Could you check a few things on this model? Use its own coordinates, in mm. A direction names the side the tool comes from. Coordinates: 2 decimals unless noted, no trailing zeros. Write each loop counter-clockwise with the first axis right and the second up, starting at its lowest first coordinate (ties: lowest second). Pieces come first, ordered by that corner, then holes. Notation, with made-up numbers: M -3,17.25 L 16,17.25 A22 ccw 16,28.25 Z; hole C 43.25,31.25 d8. An arc over 180 degrees is marked long. Answer as CSV lines item,"result". Start each with the question number.
Item 1: I'm going to push flat-ended pins straight in: P1, Ø3, axis at y = 8.5, z = -17, coming from the +X side; P2, Ø4, axis at x = -25.5, z = 30.5, coming from the +Y side; P3, Ø1.7, axis at x = 20, z = 26.5, coming from the -Y side; P4, Ø3.5, axis at x = 31.5, z = -10, coming from the -Y side. Where does each tip first touch, or does it pass through?
Item 2: If I drill on line 1 along X through (y, z) = (10.4, 0); line 2 along Y through (x, z) = (-27, 0), over which ranges is the centre line in solid material (lowest first)? Write a range as [from, to].
Item 3: We'd pull the mould along Z, two halves only. Please class faces 1 (the flat face through (0, 11.7, -33)), 2 (the flat face through (-1, 16.5, -1)), 3 (the cylindrical face through (-5.077, 8.134, -38.668)): +Z half, -Z half, draft (parallel to the pull), parting line (faces both ways), or undercut.
Item 4: Suppose I cut it at A-A, the plane x = 0. Write out the boundary of the cut face in (y, z), and give its area (3 significant figures).
Item 5: Suppose I cut it at B-B, the plane y = 10.5. Write out the boundary of the cut face in (x, z).
Item 6: Suppose I cut it at D-D, the plane y = 4.75. Write out the boundary of the cut face in (x, z), and give its area (3 significant figures).
Item 7: On a 3-axis mill with a long thin cutter (end or side, diameter ignored), from which of +Z, -Z, +X, -X, +Y, -Y can I reach the whole of each face in a straight line? I mean faces 4 (the flat face through (11.4, 0, 34.5)), 5 (the flat face through (19, 11.7, 27)). Say none if no direction works.
Item 8: Suppose I cut it at C-C, the plane z = -2. Write out the boundary of the cut face in (x, y).
```python
from build123d import *

# Parameters (mm, degrees)
SKETCH1_R           = 39
SKETCH1_R_2         = 36
BOSS_EXTRUDE2_DEPTH = 8.5
SKETCH2_R           = 39
SKETCH2_R_2         = 30
SKETCH2_R_3         = 1.698645883
BOSS_EXTRUDE3_DEPTH = 3.2
SKETCH4_R           = 39
SKETCH4_R_2         = 30
BOSS_EXTRUDE6_DEPTH = 2.8
SKETCH11_R          = 39
BOSS_EXTRUDE7_DEPTH = 2


with BuildPart() as part:
    # Sketch1 → Boss-Extrude2 (new body)
    with BuildSketch(Plane(origin=(0, 0, 0), x_dir=(1, 0, 0), z_dir=(0, 1, 0))):
        Circle(SKETCH1_R)
        Circle(SKETCH1_R_2, mode=Mode.SUBTRACT)
    extrude(amount=BOSS_EXTRUDE2_DEPTH)

    # Sketch2 → Boss-Extrude3 (add)
    with BuildSketch(Plane(origin=(0, 8.5, 0), x_dir=(1, 0, 0), z_dir=(0, 1, 0))):
        Circle(SKETCH2_R)
        Circle(SKETCH2_R_2, mode=Mode.SUBTRACT)
        with Locations((0, 33)):
            Circle(SKETCH2_R_3, mode=Mode.SUBTRACT)
        with Locations((31.384865038, 10.197560814)):
            Circle(SKETCH2_R_3, mode=Mode.SUBTRACT)
        with Locations((19.396913326, -26.697560814)):
            Circle(SKETCH2_R_3, mode=Mode.SUBTRACT)
        with Locations((-19.396913326, -26.697560814)):
            Circle(SKETCH2_R_3, mode=Mode.SUBTRACT)
        with Locations((-31.384865038, 10.197560814)):
            Circle(SKETCH2_R_3, mode=Mode.SUBTRACT)
    extrude(amount=BOSS_EXTRUDE3_DEPTH)

    # Sketch4 → Boss-Extrude6 (add)
    with BuildSketch(Plane(origin=(0, 11.7, 0), x_dir=(1, 0, 0), z_dir=(0, 1, 0))):
        Circle(SKETCH4_R)
        Circle(SKETCH4_R_2, mode=Mode.SUBTRACT)
    extrude(amount=BOSS_EXTRUDE6_DEPTH)

    # Sketch11 → Boss-Extrude7 (add)
    with BuildSketch(Plane(origin=(0, 14.5, 0), x_dir=(1, 0, 0), z_dir=(0, 1, 0))):
        Circle(SKETCH11_R)
    extrude(amount=BOSS_EXTRUDE7_DEPTH)


solid = part.part
```
Ans:
1,P1,"stops at x = 35.79"
1,P2,"stops at y = 16.5"
1,P3,"stops at y = 11.7"
1,P4,"stops at y = 8.5"
2,line 1,"x = [-39, -30], [30, 39]"
2,line 2,"y = [14.5, 16.5]"
3,face 1,"undercut"
3,face 2,"draft"
3,face 3,"parting line"
4,outline,"M 0,-39 L 16.5,-39 L 16.5,39 L 0,39 L 0,36 L 8.5,36 L 8.5,30 L 14.5,30 L 14.5,-30 L 8.5,-30 L 8.5,-31.3 L 11.7,-31.3 L 11.7,-34.7 L 8.5,-34.7 L 8.5,-36 L 0,-36 Z"
4,area,"304 mm^2"
5,outline,"C 0,0 d78; hole C -31.38,-10.2 d3.4; hole C 0,0 d60; hole C -19.4,26.7 d3.4; hole C 0,-33 d3.4; hole C 19.4,26.7 d3.4; hole C 31.38,-10.2 d3.4"
6,outline,"C 0,0 d78; hole C 0,0 d72"
6,area,"707 mm^2"
7,face 4,"+Z, -Z, +X, -X, -Y"
7,face 5,"-Y"
8,outline,"M -38.95,0 L -35.94,0 L -35.94,8.5 L -29.93,8.5 L -29.93,14.5 L 29.93,14.5 L 29.93,8.5 L 35.94,8.5 L 35.94,0 L 38.95,0 L 38.95,16.5 L -38.95,16.5 Z"
